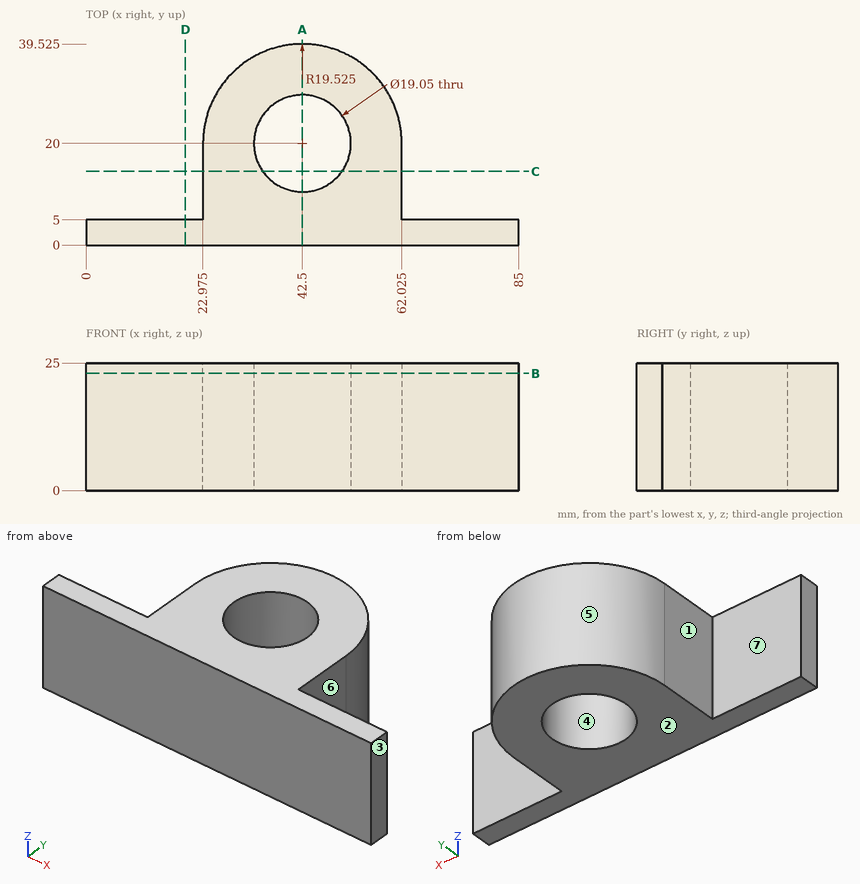
Source: three-view drawing plus pictorial views. Frame: mm from the lowest corner of the part. A direction names the side the tool comes from. Coordinates: 2 decimals unless noted, no trailing zeros. Loops run counter-clockwise (first coordinate to the right, second up) from the corner with the lowest first, then second, coordinate; pieces in that order, holes last. Notation, with made-up numbers: (81.25, 17) - (136.25, 17) arc R17 ccw to (136.25, 28) - close; hole circle Ø1 at (88.5, 64). An arc over 180 degrees is marked (long way). Answer in a Markdown table with one row per item. Add a question column.
Item 1: Section query B-B on z = 23. Return the cut outline in (x, y) (3 decimals), then the cut area to 3 significant figures.
Item 2: Access query for the marked faces 5, 6 and 7. Directions: +Z, -Z, +X, -X, +Y, -Y. A direction counts if a zero-diameter tool reaches every point of the face in a straight line with its end or side. Return the directions, or none.
Item 3: Mould query, pull axis X, two halves, no side actions, for the marked faces 1, 2, 3 and 4. Classes: released by +X, released by -X, zero draft, split by the parting line, or undercut.
Item 4: Section query A-A on x = 42.5. Return the cut outline in (y, z) (3 decimals), then the cut area to 3 significant figures.
Item 5: Line query: line 1 along Y through (x, z) = (42.5, 6.5) (3 decimals); line 2 along Y through (x, z) = (76, 12.25); line 3 along X through (y, z) = (17, 10.5) (3 decimals). Output: solid intervals per line, ascending. Write a range as [from, to].
Item 6: Section query D-D on x = 19.5. Return the cut outline in (y, z), then the cut area to 3 significant figures.
Item 7: Contact query for flat-ended pins moving along their axis: P1, Ø1.5, axis at y = 19, z = 14, coming from the -X side (3 decimals); P2, Ø15, axis at x = 42.5, y = 20, coming from the -Z side; P3, Ø1, axis at x = 24.5, z = 7.5, coming from the +Y side; P4, Ø3, axis at y = 26.5, z = 19, coming from the +X side. Output: stop coordinate, or through.
Item 8: Section query C-C on y = 14.5. Return the cut outline in (x, z) (3 decimals).
Recorded:
| question | item | result |
|---|---|---|
| 1 | outline | (0, 0) - (85, 0) - (85, 5) - (62.025, 5) - (62.025, 20) arc R19.525 ccw to (22.975, 20) - (22.975, 5) - (0, 5) - close; hole circle Ø19.05 at (42.5, 20) |
| 1 | area | 1,320 mm^2 |
| 2 | face 5 | +Z, -Z, +Y |
| 2 | face 6 | +Z, -Z, +X, +Y |
| 2 | face 7 | +Z, -Z, -X, +Y |
| 3 | face 1 | released by -X |
| 3 | face 2 | zero draft |
| 3 | face 3 | released by +X |
| 3 | face 4 | undercut |
| 4 | outline | (0, 0) - (10.475, 0) - (10.475, 25) - (0, 25) - close; (29.525, 0) - (39.525, 0) - (39.525, 25) - (29.525, 25) - close |
| 4 | area | 512 mm^2 |
| 5 | line 1 | [0, 10.475], [29.525, 39.525] |
| 5 | line 2 | [0, 5] |
| 5 | line 3 | [22.975, 33.46], [51.54, 62.025] |
| 6 | outline | (0, 0) - (5, 0) - (5, 25) - (0, 25) - close |
| 6 | area | 125 mm^2 |
| 7 | P1 | x = 22.975 |
| 7 | P2 | through |
| 7 | P3 | y = 28.66 |
| 7 | P4 | x = 61.37 |
| 8 | outline | (22.975, 0) - (34.723, 0) - (34.723, 25) - (22.975, 25) - close; (50.277, 0) - (62.025, 0) - (62.025, 25) - (50.277, 25) - close |
